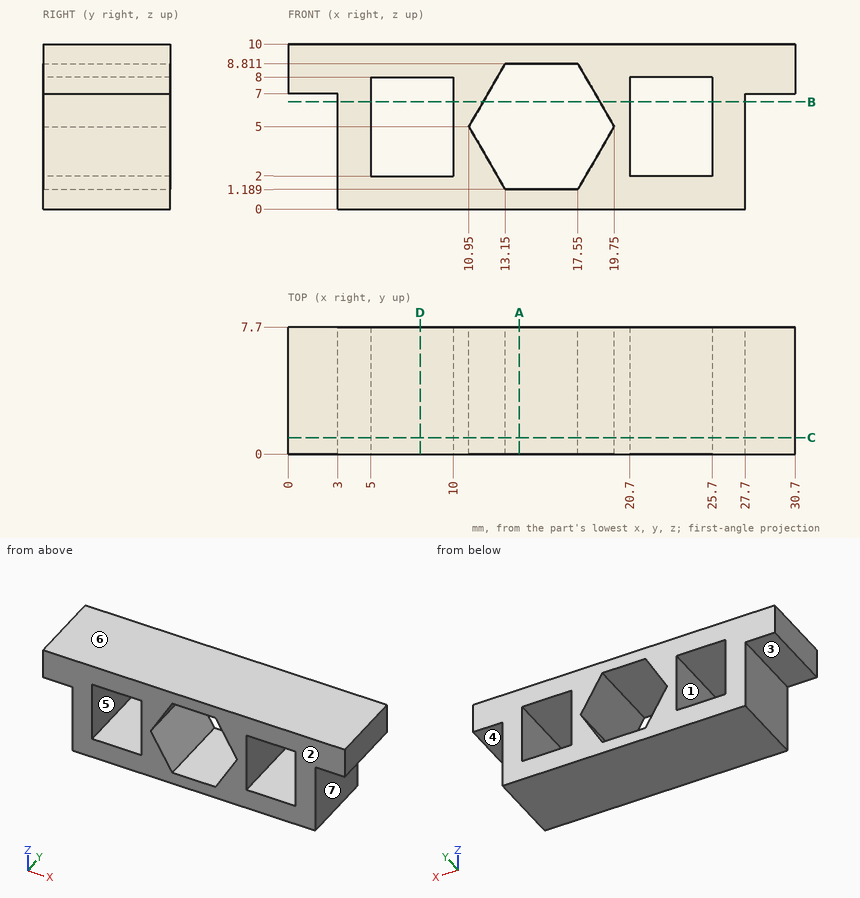
Source: three-view drawing plus pictorial views. Frame: mm from the lowest corner of the part. A direction names the side the tool comes from. Round coordinates to 2 decimals unless told otherwise and drop trailing zeros. Loops run counter-clockwise (first coordinate to the right, second up) from the corner with the lowest first, then second, coordinate; pieces in that order, holes last. Notation, with made-up numbers: (20, -1) - (57, -1) arc R5 cw to (57, 8) - close; hole circle Ø7 at (43.25, 24). An arc over 180 degrees is marked (long way). Write item = value, one per line. Start each with the question number.
Item 1: Reachability of the marked faces 1, 2, 3 and 4 from +Z, -Z, +X, -X, +Y, -Y: full face, straight path, thin tool, end or side. Return the list, or none.
Item 2: Section query D-D on x = 8. Output: boundary loops of the cut face in (y, z), plus the area to 3 significant figures.
Item 3: Mould query, pull axis X, two halves, no side actions, for the marked faces 5, 6 and 7. Classes: released by +X, released by -X, zero draft, split by the parting line, or undercut.
Item 4: Section query C-C on y = 1. Output: boundary loops of the cut face in (x, z).
Item 5: Material intervals for line 1 (Z direction, x = 25.5, y = 3); line 2 (X direction, y = 4.25, z = 3) (1 decimal); line 3 (X direction, y = 0.75, z = 4.75) (1 decimal), sorted ascending.
Item 6: Section query A-A on x = 14. Output: boundary loops of the cut face in (y, z).
Item 7: First-contact query: pin 1 Ø1.8 at (y, z) = (4, 4.5) entering from +X; pin 2 Ø2 at (y, z) = (3.5, 4) entering from -X; pin 3 Ø0.9 at (x, y) = (2, 4.5) entering from -Z. Flat tips, straight axial feed; report the tip coordinate or a pass-through.
Item 8: Section query B-B on z = 6.5. Output: boundary loops of the cut face in (x, y).
Results list:
q1.face_1 = +Y, -Y
q1.face_2 = +Z, -Z, +X, -X, -Y
q1.face_3 = -Z, -X, +Y, -Y
q1.face_4 = -Z, +X, +Y, -Y
q2.outline = (0, 0) - (7.7, 0) - (7.7, 2) - (0, 2) - close; (0, 8) - (7.7, 8) - (7.7, 10) - (0, 10) - close
q2.area = 30.8 mm²
q3.face_5 = undercut
q3.face_6 = zero draft
q3.face_7 = released by +X
q4.outline = (0, 7) - (3, 7) - (3, 0) - (27.7, 0) - (27.7, 7) - (30.7, 7) - (30.7, 10) - (0, 10) - close; hole (5, 2) - (10, 2) - (10, 8) - (5, 8) - close; hole (10.95, 5) - (13.15, 1.19) - (17.55, 1.19) - (19.75, 5) - (17.55, 8.81) - (13.15, 8.81) - close; hole (20.7, 2) - (25.7, 2) - (25.7, 8) - (20.7, 8) - close
q5.line_1 = 0 to 2, 8 to 10
q5.line_2 = 3 to 5, 10 to 12.1, 18.6 to 20.7, 25.7 to 27.7
q5.line_3 = 3 to 5, 10 to 11.1, 19.6 to 20.7, 25.7 to 27.7
q6.outline = (0, 0) - (7.7, 0) - (7.7, 1.19) - (0, 1.19) - close; (0, 8.81) - (7.7, 8.81) - (7.7, 10) - (0, 10) - close
q7.pin_1 = 27.7
q7.pin_2 = 3
q7.pin_3 = 7
q8.outline = (3, 0) - (5, 0) - (5, 7.7) - (3, 7.7) - close; (10, 0) - (11.82, 0) - (11.82, 7.7) - (10, 7.7) - close; (18.88, 0) - (20.7, 0) - (20.7, 7.7) - (18.88, 7.7) - close; (25.7, 0) - (27.7, 0) - (27.7, 7.7) - (25.7, 7.7) - close
